Autodesk Inventor part; units mm, degrees
ref_plane "YZ Plane" through (0, 0, 0) normal (1, 0, 0) x (0, 1, 0)
ref_plane "XZ Plane" through (0, 0, 0) normal (0, 1, 0) x (-1, 0, 0)
ref_plane "XY Plane" through (0, 0, 0) normal (0, 0, 1) x (1, 0, 0)
sketch "Sketch_1" plane through (0, 0, 0) normal (0, 0, 1) x (1, 0, 0)
  line L0 (91, 0) -> (0, 0)
  line L1 (0, 0) -> (0, 3.5)
  line L2 (0, 3.5) -> (0.5, 4)
  line L3 (0.5, 4) -> (90.5, 4)
  line L4 (90.5, 4) -> (91, 3.5)
  line L5 (91, 3.5) -> (91, 0)
  line L6 (91, 0) -> (0, 0)
revolve "Revolution1" add sketch "Sketch_1" angle 360 about axis through (91, 0, 0) along (1, 0, 0)
sketch "Sketch2" plane through (0, 0, 0) normal (-1, 0, 0) x (0, 0, 1)
  point P0 (0, 0)
hole "Hole1" at (0, 0, 0) direction (1, 0, 0) diameter 3.242 depth 13.0641 tip angle 120 countersink diameter 4 countersink angle 90
sketch "Sketch3" plane through (91, 0, 0) normal (1, 0, 0) x (0, 0, -1)
  point P0 (0, 0)
hole "Hole2" at (91, 0, 0) direction (-1, 0, 0) diameter 3.242 depth 13.0641 tip angle 120 countersink diameter 4 countersink angle 90
properties part number "SFHRW8-91-M4-N4" material "鋼、炭素鋼"
Can you work these out from the model? Positions are in its coordinate system, mm. A direction names the side the tool comes from. Give positions to 0.01 mm unless a question says otherwise; leave off trailing zeros. Loops run counter-clockwise (first coordinate to the right, second up) from the corner with the lowest first, then second, coordinate; pieces in that order, holes last. Notation, with made-up numbers: (21.5, -29.5) - (42.5, -29.5) arc R18 ccw to (42.5, 3.5) - close; hole circle Ø5 at (-5.75, 66). An arc over 180 degrees is marked (long way). Answer as a JSON object with one key per item and string values.
Q1. Imagine slicing it at B-B on x = 23. Write out the boundary of the cut face in (y, z).
Geometry says:
{"outline": "circle Ø8 at (0, 0)"}
Q2. Will these pins go through, and if not, where does the flat tip stop? P1, Ø3.5, axis at y = 0, z = 0, coming from the -X side; P2, Ø2, axis at x = 53, y = -2.5, coming from the +Z side; P3, Ø2, axis at x = 20.5, z = -1.5, coming from the -Y side.
Geometry says:
{"P1": "x = 0.25", "P2": "z = 3.71", "P3": "y = -3.97"}
Q3. Imagine slicing it at A-A on x = 10.5. Write out the boundary of the cut face in (y, z), plus the area to 3 significant figures.
Geometry says:
{"outline": "circle Ø8 at (0, 0); hole circle Ø3.24 at (0, 0)", "area": "42.0 mm²"}
Q4. Which directions (+Z, -Z, +X, -X, +Y, -Y) give clear straight access to the entire face, cutting with the end or side of a thin tool? Please do faces 4 (the cylindrical face through (84.19, 1.438, -0.748)), 5 (the flat face through (0, 2, -2)).
Geometry says:
{"face 4": "+X", "face 5": "+Z, -Z, -X, +Y, -Y"}
Q5. If we mould it in two halves opening along Y, with no side actions, what happens to faces 1 (the flat face through (91, 2, -2)), 2 (the cylindrical face through (6.81, 1.438, 0.748)), 3 (the cylindrical face through (46.13, -0.867, -3.905))? For each: pulls with the +Y half, pulls with the -Y half, needs draft (parallel to the pull), parting line crosses it, or undercut.
Geometry says:
{"face 1": "needs draft", "face 2": "undercut", "face 3": "parting line crosses it"}
Q6. If I drill on L1, parallel to Z at x = 81.75, y = 0; L2, parallel to Y at x = 85.5, z = 1; L3, parallel to Y at x = 7, z = -3, over which ranges is the centre line in solid material (lowest first)?
Geometry says:
{"L1": "-4 to -1.62, 1.62 to 4", "L2": "-3.87 to -1.28, 1.28 to 3.87", "L3": "-2.65 to 2.65"}
